Geometry check sheet. Reference: the model listing, model coordinates, mm. A direction names the side the tool comes from. Round coordinates to 2 decimals unless told otherwise and drop trailing zeros. Loops run counter-clockwise (first coordinate to the right, second up) from the corner with the lowest first, then second, coordinate; pieces in that order, holes last. Notation, with made-up numbers: (-22, 29) - (15, 29) arc R38 cw to (15, 67) - close; hole circle Ø8 at (-25, -14). An arc over 180 degrees is marked (long way). Answer as CSV lines item,"result". Start each with the question number.
1) Cross-section at A-A on z = 8.5. Record the boundary of the cut face in (x, y).
2) Access from +Z, -Z, +X, -X, +Y, -Y to the whole of each face (thin tool, end or side, straight path). Record for faces 3 (the cylindrical face through (25.25, -0.08, 20.02)), 4 (the flat face through (4, -18, 21.5)), 5 (the flat face through (0, 0, 2)), 6 (the flat face through (-20, -1, 18.5)), 7 (the flat face through (13.5, 13, 17)).
3) Depth check by flat-ended pin: P1, Ø0.6, axis at x = 4, y = 19, coming from the +Z side; P2, Ø1, axis at x = 4, z = 12, coming from the +Y side; P3, Ø6, axis at x = -20, z = 13.5, coming from the -Y side; P4, Ø3, axis at x = 23.5, y = 0, coming from the +Z side. Enter the tip coordinate at first touch or a pass-through.
4) Draft check along X on faces 1 (the flat face through (21, 0, 18.5)), 2 (the cylindrical face through (-21.75, -0.08, 20.02)). Enter one of: released by +X, released by -X, zero draft, split by the parting line, or undercut.
5) Cross-section at B-B on z = 12. Record the boundary of the cut face in (x, y), and give its area (3 significant figures).
6) Thickness scan on line 1 along X through (y, z) = (0, 19.25); line 2 along X through (y, z) = (0, 14); line 3 along Z through (x, y) = (14.5, -13.5). Record the ranges inside material, lowest first.
Autodesk Fusion 360 part; units mm, degrees
sketch "Sketch1" plane through (0, 0, 0) normal (0, 0, 1) x (1, 0, 0)
  circle A0 centre (0, 0) radius 19.75
  dimension "d1" = 39.5
extrude "Extrude1" add sketch "Sketch1" along normal blind 2
sketch "Sketch2" plane through (0, 0, 2) normal (0, 0, 1) x (-1, 0, 0)
  circle A0 centre (0, 0) radius 19.75
  circle A1 centre (0, 0) radius 11.75
  circle A2 centre (0, 0) radius 19.75
  dimension "d4" = 23.5
extrude "Extrude2" add sketch "Sketch2" along normal blind 7.5
sketch "Sketch3" plane through (0, 0, 9.5) normal (0, 0, 1) x (-1, 0, 0)
  circle A0 centre (0, 0) radius 11.75
  circle A1 centre (0, 0) radius 19.75
  circle A2 centre (0, 0) radius 19.75
  circle A3 centre (0, 0) radius 18
  dimension "d7" = 36
extrude "Extrude3" add sketch "Sketch3" along normal blind 12 contours A1 A2
sketch "Sketch4" plane through (0, 0, 21.5) normal (0, 0, 1) x (-1, 0, 0)
  circle A0 centre (0, 0) radius 18
  circle A1 centre (0, 0) radius 19.75
  circle A2 centre (0, 0) radius 19.75
  line L0 (-27, -19.75) -> (27, -19.75)
  line L1 (27, -19.75) -> (27, 19.75)
  line L2 (27, 19.75) -> (-27, 19.75)
  line L3 (-27, 19.75) -> (-27, -19.75)
  line L4 (-27, -19.75) -> (27, 19.75) construction
  line L5 (27, -19.75) -> (-27, 19.75) construction
  line L6 (-27, 0) -> (-23.5, 0)
  line L7 (27, 0) -> (23.5, 0)
  circle A3 centre (23.5, 0) radius 1.75
  circle A4 centre (-23.5, 0) radius 1.75
  dimension "d10" = 39.5
  dimension "d11" = 54
  dimension "d12" = 3.5
  dimension "d13" = 3.5
  dimension "d14" = 3.5
  dimension "d15" = 3.5
extrude "Extrude4" add sketch "Sketch4" against normal blind 3 contours A1 A2 L0 L1 L2 | A1 A2 L0 L2 L3
sketch "Sketch5" plane through (0, 0, 21.5) normal (0, 0, 1) x (-1, 0, 0)
  circle A0 centre (23.5, 0) radius 1.75
  circle A1 centre (-23.5, 0) radius 1.75
  circle A2 centre (0, 0) radius 18
  line L0 (-27, -19.75) -> (27, -19.75)
  line L1 (27, -19.75) -> (27, 19.75)
  line L2 (27, 19.75) -> (-27, 19.75)
  line L3 (-27, 19.75) -> (-27, -19.75)
  ellipse E0 centre (0, 0) end of major axis (-27, 0) minor radius 19.75
  line L4 (27, 0) -> (-27, 0) construction
  line L5 (0, 19.75) -> (0, -19.75) construction
  line L6 (27, -19.75) -> (-27, -19.75)
  line L7 (-27, -19.75) -> (-27, 19.75)
  line L8 (-27, 19.75) -> (27, 19.75)
  line L9 (27, 19.75) -> (27, -19.75)
extrude "Extrude5" cut sketch "Sketch5" against normal blind 10 contours L0 L3 E0 L6 L7 | L0 L1 E0 L6 L9 | L2 L3 E0 L7 L8 | L1 L2 E0 L8 L9
ref_plane "WorkPlane1" through (0, 11.75, 7.4179) normal (0, -1, 0) x (-1, 0, 0)
ref_plane "WorkPlane2" through (0, 17.75, 7.4179) normal (0, -1, 0) x (-1, 0, 0)
sketch "Sketch6" plane through (0, 17.75, 0) normal (0, -1, 0) x (-1, 0, 0)
  line L0 (0, 0) -> (0, -15.5)
  line L1 (-30, -21.5) -> (30, -21.5)
  line L2 (30, -21.5) -> (30, -9.5)
  line L3 (30, -9.5) -> (-30, -9.5)
  line L4 (-30, -9.5) -> (-30, -21.5)
  line L5 (-30, -21.5) -> (30, -9.5) construction
  line L6 (30, -21.5) -> (-30, -9.5) construction
  line L7 (30, -21.5) -> (-30, -21.5)
  line L8 (-30, -21.5) -> (-30, -35.9601)
  line L9 (-30, -35.9601) -> (30, -35.9601)
  line L10 (30, -35.9601) -> (30, -21.5)
  point P0 (0, -15.5)
  dimension "d22" = 15.5
  dimension "d23" = 12
  dimension "d24" = 60
  dimension "d25" = 60
extrude "Extrude6" cut sketch "Sketch6" against normal blind 20
sketch "Sketch7" plane through (0, 17.75, 0) normal (0, 1, 0) x (-1, 0, 0)
  line L0 (-8.6603, 18.5) -> (-8.6603, 9.5)
  line L1 (-8.6603, 9.5) -> (-2.9896, 9.5)
  line L2 (-2.9896, 9.5) -> (-2.9896, 21.5)
  line L3 (-2.9896, 21.5) -> (-11.8393, 21.5)
  line L4 (-11.8393, 21.5) -> (-11.8393, 18.5)
  line L5 (-11.8393, 18.5) -> (-8.6603, 18.5)
  line L6 (13.5, 23.7273) -> (-13.5, 23.7273)
  line L7 (-13.5, 23.7273) -> (-13.5, -4.7273)
  line L8 (-13.5, -4.7273) -> (13.5, -4.7273)
  line L9 (13.5, -4.7273) -> (13.5, 23.7273)
  line L10 (13.5, 23.7273) -> (-13.5, -4.7273) construction
  line L11 (-13.5, 23.7273) -> (13.5, -4.7273) construction
  line L12 (0, 9.5) -> (13.5, 9.5)
  line L13 (0, 9.5) -> (-13.5, 9.5)
  point P0 (0, 9.5)
  dimension "d28" = 27
extrude "Extrude7" cut sketch "Sketch7" against normal blind 20 contours L0 L1 L2 L3 L4 L5 L13 | L0 L2 L3 L4 L5 L6 L7 L9 L12 L13
Answer block:
1,outline,"circle Ø39.5 at (0, 0); hole circle Ø23.5 at (0, 0)"
2,face 3,"+Z, -Z"
2,face 4,"+Z, +X, -X, +Y, -Y"
2,face 5,"+Z"
2,face 6,"-Z, -X"
2,face 7,"+Z, +Y"
3,P1,"stops at z = 9.5"
3,P2,"stops at y = -17.43"
3,P3,"stops at y = -10.05"
3,P4,"passes through"
4,face 1,"zero draft"
4,face 2,"undercut"
5,outline,"(-13.5, 11.91) - (-13.5, 14.42) arc R19.75 ccw (long way) to (13.5, 14.42) - (13.5, 11.91) arc R18 cw (long way) to start"
5,area,"155 mm^2"
6,line 1,"x = -27 to -25.25, -21.75 to -18, 18 to 21.75, 25.25 to 27"
6,line 2,"x = -19.75 to -18, 18 to 19.75"
6,line 3,"z = 18.5 to 21.5"
